The listing builds one solid part. Answer for the finished solid, in the listing's coordinates (mm). Round coordinates to 2 decimals unless told otherwise and drop trailing zeros. Order: outer loops, then holes, each group sorted by start corner. A loop starts at its lowest first (then second) coordinate and runs counter-clockwise, first axis right, second up. Notation, with made-up numbers: M -1,2 L 23,2 A24 ccw 23,39 Z; hole C 50,40.25 d7. An arc over 180 degrees is marked long. Put each result on its own line as item: value. Start each with the question number.
1. The part is cut by section A-A (y = -1.25). Give the vertices of the cut face in (x, z), then the cut area to 3 significant figures.
2. Consider line 1 (X direction, y = 1, z = -88.5); line 2 (Z direction, x = -50.8, y = 2.75); line 3 (X direction, y = -2.5, z = 90.5). Determine where each line is inside the solid, lowest interval first.
3. The part is cut by section C-C (x = 96). Give the vertices of the cut face in (y, z).
4. The part is cut by section B-B (z = -25.5). Give the vertices of the cut face in (x, y), then the cut area to 3 significant figures.
5. Each of these flat-tipped pins is pushed along its axis until it touches: pin 1 Ø1 at (x, y) = (70.5, -3) entering from -Z; pin 2 Ø3 at (x, y) = (-79, 3.5) entering from -Z; pin 3 Ø14.5 at (x, z) = (105, -1.96) entering from +Y; pin 4 Ø1 at (y, z) = (-1.5, -13.5) entering from +X. Where does it stop, or does it pass through?
from build123d import *

# Parameters (mm, degrees)
BOSS_EXTRUDE1_DEPTH = 4.7625
SKETCH2_R           = 5.55625
CUT_EXTRUDE1_DEPTH  = 10.525
CIRPATTERN1_COUNT   = 3


with BuildPart() as part:
    # Sketch1 → Boss-Extrude1 (new body, symmetric)
    with BuildSketch(Plane(origin=(0, 0, 0), x_dir=(1, 0, 0), z_dir=(0, 1, 0))):
        Polygon((-50.8, 146.646968374), (50.8, 146.646968374), (152.4, -29.329393675), (101.6, -117.317574699), (-101.6, -117.317574699), (-152.4, -29.329393675), align=None)
    extrude(amount=BOSS_EXTRUDE1_DEPTH, both=True)

    # Sketch2 → Cut-Extrude1 (cut, through all)
    with BuildSketch(Plane(origin=(0, 4.7625, 0), x_dir=(1, 0, 0), z_dir=(0, 1, 0))):
        with Locations((105.002954744, 1.964696837)):
            Circle(SKETCH2_R)
        with Locations((54.202954744, 89.952877862)):
            Circle(SKETCH2_R)
    cut_extrude1 = extrude(amount=-CUT_EXTRUDE1_DEPTH, mode=Mode.SUBTRACT)

    # CirPattern1: Cut-Extrude1 ×3 about axis
    cirpattern1_axis = Axis((0, 0, 0), (0, 1, 0))
    for i in range(1, CIRPATTERN1_COUNT):
        add(cut_extrude1.rotate(cirpattern1_axis, i * 360 / CIRPATTERN1_COUNT), mode=Mode.SUBTRACT)


solid = part.part
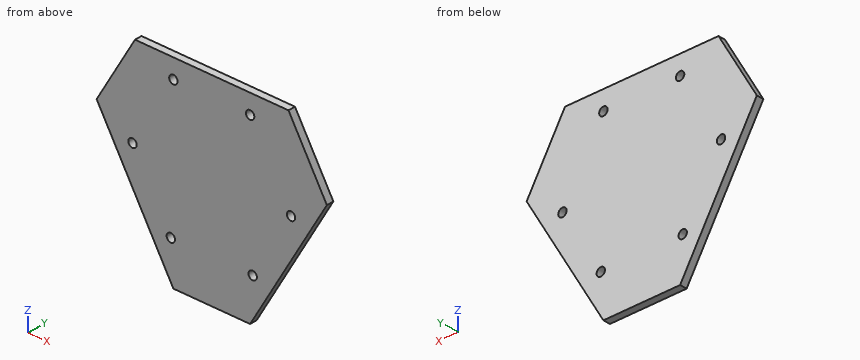
Resolved:
1. outline: M -152.4,29.33 L -50.8,-146.65 L 50.8,-146.65 L 152.4,29.33 L 101.6,117.32 L -101.6,117.32 Z; hole C -105,-1.96 d11.11; hole C -54.2,-89.95 d11.11; hole C -50.8,91.92 d11.11; hole C 50.8,91.92 d11.11; hole C 54.2,-89.95 d11.11; hole C 105,-1.96 d11.11
1. area: 57,500 mm2
2. line 1: -84.37 to -59.57, -48.84 to 48.84, 59.57 to 84.37
2. line 2: -146.65 to -94.35, -85.56 to 86.36, 97.47 to 117.32
2. line 3: -117.08 to -56.17, -45.43 to 45.43, 56.17 to 117.08
3. outline: M -4.76,-68.36 L 4.76,-68.36 L 4.76,117.32 L -4.76,117.32 Z
4. outline: M -120.74,-4.76 L 120.74,-4.76 L 120.74,4.76 L -120.74,4.76 Z
4. area: 2,300 mm2
5. pin 1: z = -113.39
5. pin 2: z = -100.4
5. pin 3: y = 4.76
5. pin 4: x = 127.96
